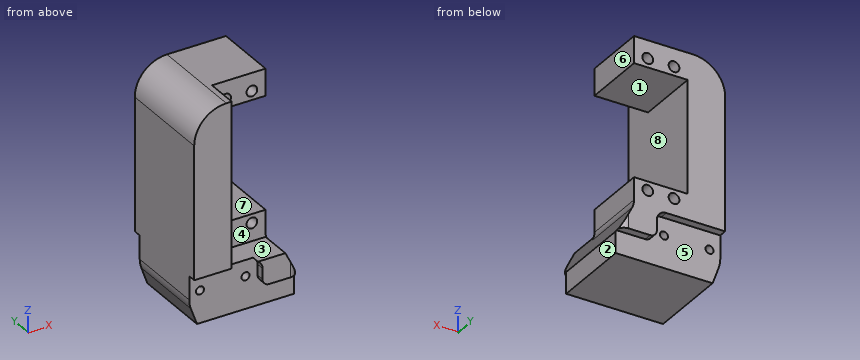
from build123d import *

# Parameters (mm, degrees)
BOSS_EXTRUDE1_DEPTH     = 36
CUT_EXTRUDE2_DEPTH      = 3
CUT_EXTRUDE3_DEPTH      = 3
FILLET3_R               = 12
SKETCH5_W               = 25.000013064
SKETCH5_H               = 10
SKETCH5_H_2             = 9.999999996
CUT_EXTRUDE4_DEPTH      = 12
CUT_EXTRUDE5_DEPTH      = 13
CUT_EXTRUDE5_DEPTH_BACK = 25
FILLET4_R               = 7
CUT_EXTRUDE6_DEPTH      = 1
CUT_EXTRUDE6_DEPTH_BACK = 81
SKETCH8_R               = 1.5
SKETCH8_R_2             = 2
CUT_EXTRUDE7_DEPTH      = 34


with BuildPart() as part:
    # Sketch1 → Boss-Extrude1 (new body)
    with BuildSketch(Plane.XZ.offset(-33.496710387)):
        with BuildLine():
            Line((-28.572528903, 54.343907724), (-28.572528903, 64.34390772))
            Line((-28.572528903, 64.34390772), (-67.573393535, 64.34390772))
            Line((-67.573393535, 64.34390772), (-67.573393535, -5.916364341))
            ThreePointArc((-67.573393535, -5.916364341), (-67.425411698, -7.63034746), (-66.98584591, -9.293602903))
            Line((-66.98584591, -9.293602903), (-64.702950485, -15.65609228))
            Line((-64.702950485, -15.65609228), (-28.572528903, -15.65609228))
            Line((-28.572528903, -15.65609228), (-28.572528903, 12.343907724))
            Line((-28.572528903, 12.343907724), (-53.572541967, 12.343907724))
            Line((-53.572541967, 12.343907724), (-53.572541967, 54.343907724))
            Line((-53.572541967, 54.343907724), (-28.572528903, 54.343907724))
        make_face()
    extrude(amount=BOSS_EXTRUDE1_DEPTH)

    # Sketch3 → Cut-Extrude2 (cut)
    with BuildSketch(Plane.XZ.offset(2.503289613)):
        with BuildLine():
            Line((-28.572528903, -15.65609228), (-67.573393527, -15.65609228))
            Line((-67.573393527, -15.65609228), (-67.573393527, 2.843907727))
            Line((-67.573393527, 2.843907727), (-45.573393535, 2.843907727))
            ThreePointArc((-45.573393535, 2.843907727), (-43.098519801, 1.818781461), (-42.073393535, -0.656092273))
            Line((-42.073393535, -0.656092273), (-42.073393535, -4.656092274))
            ThreePointArc((-42.073393535, -4.656092274), (-41.341160488, -6.423859227), (-39.573393535, -7.156092274))
            Line((-39.573393535, -7.156092274), (-28.572528903, -7.156092274))
            Line((-28.572528903, -7.156092274), (-28.572528903, -15.65609228))
        make_face()
    extrude(amount=-CUT_EXTRUDE2_DEPTH, mode=Mode.SUBTRACT)

    # Sketch4 → Cut-Extrude3 (cut)
    with BuildSketch(Plane(origin=(0, 33.496710387, 0), x_dir=(1, 0, 0), z_dir=(0, 1, 0))):
        with BuildLine():
            Line((-67.573393527, 15.65609228), (-67.573393527, -2.843907727))
            Line((-67.573393527, -2.843907727), (-45.573393535, -2.843907727))
            ThreePointArc((-45.573393535, -2.843907727), (-43.098519801, -1.818781461), (-42.073393535, 0.656092273))
            Line((-42.073393535, 0.656092273), (-42.073393535, 4.656092274))
            ThreePointArc((-42.073393535, 4.656092274), (-41.341160488, 6.423859227), (-39.573393535, 7.156092274))
            Line((-39.573393535, 7.156092274), (-28.572528903, 7.156092274))
            Line((-28.572528903, 7.156092274), (-28.572528903, 15.65609228))
            Line((-28.572528903, 15.65609228), (-67.573393527, 15.65609228))
        make_face()
    extrude(amount=-CUT_EXTRUDE3_DEPTH, mode=Mode.SUBTRACT)

    # Fillet3
    fillet3_edges = [part.edges().sort_by_distance(p)[0] for p in [
        (-67.573393535, 15.496710387, 64.34390772),
    ]]
    fillet(fillet3_edges, radius=FILLET3_R)

    # Sketch5 → Cut-Extrude4 (cut)
    with BuildSketch(Plane.XZ.offset(2.503289613)):
        with Locations((-41.072535435, 7.343907724)):
            Rectangle(SKETCH5_W, SKETCH5_H)
        with Locations((-41.072535435, 59.343907722)):
            Rectangle(SKETCH5_W, SKETCH5_H_2)
    extrude(amount=-CUT_EXTRUDE4_DEPTH, mode=Mode.SUBTRACT)

    # Sketch6 → Cut-Extrude5 (cut, two sides)
    with BuildSketch(Plane.XZ.offset(-9.496710387)) as cut_extrude5_sk:
        Polygon((-33.572541967, 64.34390772), (-33.572541967, 2.343907724), (-28.572528903, -7.656092278), (-28.572528903, 64.34390772), align=None)
    extrude(amount=CUT_EXTRUDE5_DEPTH, mode=Mode.SUBTRACT)
    extrude(cut_extrude5_sk.sketch, amount=-CUT_EXTRUDE5_DEPTH_BACK, mode=Mode.SUBTRACT)

    # Fillet4
    fillet4_edges = [part.edges().sort_by_distance(p)[0] for p in [
        (-33.572541967, 21.496710387, 2.343907724),
    ]]
    fillet(fillet4_edges, radius=FILLET4_R)

    # Sketch7 → Cut-Extrude6 (cut, two sides)
    with BuildSketch(Plane(origin=(0, 0, -15.65609228), x_dir=(-1, 0, 0), z_dir=(0, 0, -1))) as cut_extrude6_sk:
        with BuildLine():
            Line((31.572528926, -2.503289613), (28.572528926, -2.503289613))
            Line((28.572528926, -2.503289613), (28.572528926, 0.496710387))
            ThreePointArc((28.572528926, 0.496710387), (29.451208582, -1.624609954), (31.572528926, -2.503289613))
        make_face()
        with BuildLine():
            Line((31.572528902, 33.496710387), (28.572528902, 33.496710387))
            Line((28.572528902, 33.496710387), (28.572528902, 30.496710387))
            ThreePointArc((28.572528902, 30.496710387), (29.451208558, 32.618030731), (31.572528902, 33.496710387))
        make_face()
    extrude(amount=CUT_EXTRUDE6_DEPTH, mode=Mode.SUBTRACT)
    extrude(cut_extrude6_sk.sketch, amount=-CUT_EXTRUDE6_DEPTH_BACK, mode=Mode.SUBTRACT)

    # Sketch8 → Cut-Extrude7 (cut, through all)
    with BuildSketch(Plane.XZ.offset(-0.496710387)):
        with Locations((-46.573393534, -3.65609228)):
            Circle(SKETCH8_R)
        with Locations((-63.573393534, -3.656092278)):
            Circle(SKETCH8_R)
        with Locations((-38.672541967, 9.043907724)):
            Circle(SKETCH8_R_2)
        with Locations((-48.472541967, 9.043907724)):
            Circle(SKETCH8_R_2)
        with Locations((-48.472541967, 57.643907724)):
            Circle(SKETCH8_R_2)
        with Locations((-38.672541967, 57.643907724)):
            Circle(SKETCH8_R_2)
    extrude(amount=-CUT_EXTRUDE7_DEPTH, mode=Mode.SUBTRACT)


solid = part.part
Verification items for the finished model (mm, model axes). Face numbers are marked on the shaded views. A direction names the side the tool comes from. Round coordinates to 2 decimals unless told otherwise and drop trailing zeros. Loops run counter-clockwise (first coordinate to the right, second up) from the corner with the lowest first, then second, coordinate; pieces in that order, holes last. Notation, with made-up numbers: (-21, 32) - (-14, 32) arc R20 cw to (-14, 58) - close; hole circle Ø9 at (57, -6). An arc over 180 degrees is marked (long way). Use a Markdown table: item, result. Add a question column.
1. Gauge pin test, flat ends, axial feed: pin 1 (3 mm diameter, centred on x = -48.47, z = 9.04, fed in from -Y); pin 2 (3.5 mm diameter, centred on x = -44.5, z = 4, fed in from -Y); pin 3 (0.9 mm diameter, centred on x = -35, y = -1, fed in from -Z); pin 4 (1.5 mm diameter, centred on y = -1.5, z = -2, fed in from -X). Record the tip position at first contact, or that the pin passes through.
2. Section check B-B, the plane x = -43. Record the boundary of the cut face in (y, z), plus the area to 3 significant figures.
3. Release check for a two-part mould opening along Z. For the marked faces 1, 2 and 3 record: released by +Z, released by -Z, zero draft, split by the parting line, or undercut.
4. Section check D-D, the plane z = 46.5. Record the boundary of the cut face in (x, y), plus the area to 3 significant figures.
5. Section check C-C, the plane y = 5. Record the boundary of the cut face in (x, z), plus the area to 3 significant figures.
6. Access from +Z, -Z, +X, -X, +Y, -Y to the whole of each face (thin tool, end or side, straight path). Record for the marked faces 4, 5, 6, 7 and 8.
7. Thickness scan on probe 1 along Z at (x, y) = (-34.5, 29); probe 2 along Z at (x, y) = (-40, 26); probe 3 along X at (y, z) = (23.5, 8). Record the ranges inside material, lowest first. Write a range as [from, to].
8. Section check A-A, the plane y = 16.5. Record the boundary of the cut face in (x, z), plus the area to 3 significant figures.
Checks:
| question | item | result |
|---|---|---|
| 1 | pin 1 | passes through |
| 1 | pin 2 | stops at y = 0.5 |
| 1 | pin 3 | stops at z = -7.16 |
| 1 | pin 4 | stops at x = -42.07 |
| 2 | outline | (-2.5, 1.72) - (0.5, 1.72) - (0.5, -15.66) - (30.5, -15.66) - (30.5, 1.72) - (33.5, 1.72) - (33.5, 12.34) - (9.5, 12.34) - (9.5, 2.34) - (-2.5, 2.34) - close; (9.5, 54.34) - (33.5, 54.34) - (33.5, 64.34) - (9.5, 64.34) - close |
| 2 | area | 1,020 mm^2 |
| 3 | face 1 | undercut |
| 3 | face 2 | zero draft |
| 3 | face 3 | released by +Z |
| 4 | outline | (-67.57, -2.5) - (-53.57, -2.5) - (-53.57, 33.5) - (-67.57, 33.5) - close |
| 4 | area | 504 mm^2 |
| 5 | outline | (-67.57, -5.92) arc R10 ccw to (-66.99, -9.29) - (-64.7, -15.66) - (-28.57, -15.66) - (-28.57, -7.66) - (-33.57, 2.34) - (-53.57, 2.34) - (-53.57, 64.34) - (-55.57, 64.34) arc R12 ccw to (-67.57, 52.34) - close; hole circle Ø3 at (-63.57, -3.66); hole circle Ø3 at (-46.57, -3.66) |
| 5 | area | 1,490 mm^2 |
| 6 | face 4 | +Z, +X, -Y |
| 6 | face 5 | -Z, -X, +Y |
| 6 | face 6 | +Z, +X, +Y, -Y |
| 6 | face 7 | +X, +Y, -Y |
| 6 | face 8 | +X, -Y |
| 7 | probe 1 | z = [-15.66, 12.34], [54.34, 64.34] |
| 7 | probe 2 | z = [-15.66, 7.55], [10.54, 12.34], [54.34, 56.15], [59.14, 64.34] |
| 7 | probe 3 | x = [-67.57, -50.18], [-46.77, -40.38], [-36.97, -33.57] |
| 8 | outline | (-67.57, -5.92) arc R10 ccw to (-66.99, -9.29) - (-64.7, -15.66) - (-28.57, -15.66) - (-28.57, -7.66) - (-32.83, 0.87) arc R7 cw to (-33.57, 4) - (-33.57, 12.34) - (-53.57, 12.34) - (-53.57, 54.34) - (-33.57, 54.34) - (-33.57, 64.34) - (-55.57, 64.34) arc R12 ccw to (-67.57, 52.34) - close; hole circle Ø3 at (-63.57, -3.66); hole circle Ø4 at (-48.47, 9.04); hole circle Ø4 at (-48.47, 57.64); hole circle Ø3 at (-46.57, -3.66); hole circle Ø4 at (-38.67, 9.04); hole circle Ø4 at (-38.67, 57.64) |
| 8 | area | 1,840 mm^2 |
